```python
from build123d import *

# Parameters (mm, degrees)
SKETCH1_R                  = 3.429
BOSS_EXTRUDE1_DEPTH        = 12.7
F_10_24_TAPPED_HOLE1_D     = 3.7973
F_10_24_TAPPED_HOLE1_DEPTH = 19.05
F_10_24_TAPPED_HOLE1_TIP   = 1.140824014


with BuildPart() as part:
    # Sketch1 → Boss-Extrude1 (new body)
    with BuildSketch(Plane.XY):
        with BuildLine():
            Line((-38.1, -17.145), (-38.1, 17.145))
            Line((-38.1, 17.145), (-22.561451151, 17.145))
            ThreePointArc((-22.561451151, 17.145), (-17.4625, 14.5796), (-12.363548849, 17.145))
            Line((-12.363548849, 17.145), (12.363548849, 17.145))
            ThreePointArc((12.363548849, 17.145), (17.4625, 14.5796), (22.561451151, 17.145))
            Line((22.561451151, 17.145), (38.1, 17.145))
            Line((38.1, 17.145), (38.1, -17.145))
            Line((38.1, -17.145), (12.7, -33.655))
            Line((12.7, -33.655), (-12.7, -33.655))
            Line((-12.7, -33.655), (-38.1, -17.145))
        make_face()
        with Locations((-17.4625, -10.795)):
            Circle(SKETCH1_R, mode=Mode.SUBTRACT)
        with Locations(Location((17.4625, -10.795, 0), (0, 0, 180))):
            Circle(SKETCH1_R, mode=Mode.SUBTRACT)
        with Locations((-17.4625, 1.905)):
            Circle(SKETCH1_R, mode=Mode.SUBTRACT)
        with Locations((0, -26.035)):
            Circle(SKETCH1_R, mode=Mode.SUBTRACT)
    extrude(amount=BOSS_EXTRUDE1_DEPTH)

    # #10-24 Tapped Hole1
    with Locations(Plane(origin=(0, 17.145, 0), x_dir=(1, 0, 0), z_dir=(0, 1, 0))):
        with Locations((-30.48, -6.35), (0, -6.35), (30.48, -6.35)):
            Hole(F_10_24_TAPPED_HOLE1_D / 2, depth=F_10_24_TAPPED_HOLE1_DEPTH)
            with Locations((0, 0, -(F_10_24_TAPPED_HOLE1_DEPTH + F_10_24_TAPPED_HOLE1_TIP / 2))):  # 118° drill point
                Cone(0, F_10_24_TAPPED_HOLE1_D / 2, F_10_24_TAPPED_HOLE1_TIP, mode=Mode.SUBTRACT)


solid = part.part
```
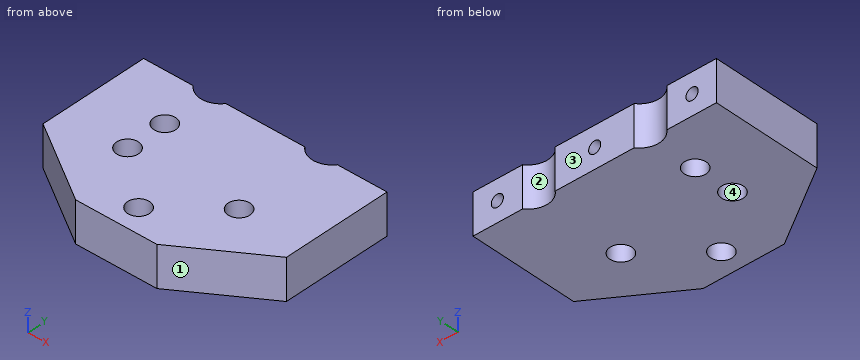
For this review, take the finished solid that the model builds, in its own axes (mm). Face numbers are marked on the shaded views. Coordinates: 2 decimals unless noted, no trailing zeros. Order: outer loops, then holes, each group sorted by start corner. A loop starts at its lowest first (then second) coordinate and runs counter-clockwise, first axis right, second up. Notation, with made-up numbers: (12.25, 35.5) - (41.25, 35.5) arc R20 cw to (41.25, 47.5) - close; hole circle Ø6 at (64, 39). An arc over 180 degrees is marked (long way). Answer as a JSON object with one key per item and string values. Group by question number.
1. Clearance check with flat-ended pins moving along their axes: P1, Ø4.5, axis at x = 30.48, z = 6.35, coming from the -Y side; P2, Ø6, axis at x = 28.5, z = 10.5, coming from the -Y side (3 decimals); P3, Ø2.5, axis at x = -30.48, z = 6.35, coming from the +Y side. State where each tip first meets the part, or that it passes through.
2. For probe 1 along X at (y, z) = (9.5, 5.25); probe 2 along Y at (x, z) = (-17, 4.5); probe 3 along Y at (x, z) = (-16, 1.5), list the stretches that pass through material, from the lowest coordinate up.
3. We need section C-C on z = 10.5. Give the number of separate pieces and of enclosed holes in the cut face, then the cut area to 3 significant figures.
4. The part is to be moulded in two halves that separate along X. For the marked faces 1, 2, 3 and 4, say which applies: pulls with the +X half, pulls with the -X half, needs draft (parallel to the pull), parting line crosses it, or undercut.
5. We need section D-D on x = 24. State the section outline as (y, z) points (3 decimals), then the cut area to 3 significant figures.
6. We need section B-B on x = -16. State the section outline as (y, z) points, then the cut area to 3 significant figures.
7. We need section A-A on y = 1. State the section outline as (x, z) points, then the cut area to 3 significant figures.
Final values:
{
 "1": {"P1": "y = -23.56", "P2": "y = -25.335", "P3": "y = -2.29"},
 "2": {"probe 1": "-38.1 to -32.03, -28.93 to -1.55, 1.55 to 28.93, 32.03 to 38.1", "probe 2": "-30.86 to -14.19, -7.4 to -1.49, 5.3 to 14.6", "probe 3": "-31.51 to -13.9, -7.69 to -1.2, 5.01 to 14.75"},
 "3": {"separate pieces": "1", "enclosed holes": "4", "area": "3,270 mm²"},
 "4": {"face 1": "pulls with the +X half", "face 2": "undercut", "face 3": "needs draft", "face 4": "undercut"},
 "5": {"outline": "(-26.31, 0) - (17.145, 0) - (17.145, 12.7) - (-26.31, 12.7) - close", "area": "552 mm²"},
 "6": {"outline": "(-31.51, 0) - (-13.9, 0) - (-13.9, 12.7) - (-31.51, 12.7) - close; (-7.69, 0) - (-1.2, 0) - (-1.2, 12.7) - (-7.69, 12.7) - close; (5.01, 0) - (14.75, 0) - (14.75, 12.7) - (5.01, 12.7) - close", "area": "430 mm²"},
 "7": {"outline": "(-38.1, 0) - (-20.77, 0) - (-20.77, 12.7) - (-38.1, 12.7) - close; (-14.16, 0) - (38.1, 0) - (38.1, 12.7) - (-14.16, 12.7) - close; hole circle Ø3.8 at (-30.48, 6.35); hole circle Ø3.8 at (0, 6.35); hole circle Ø3.8 at (30.48, 6.35)", "area": "850 mm²"}
}
